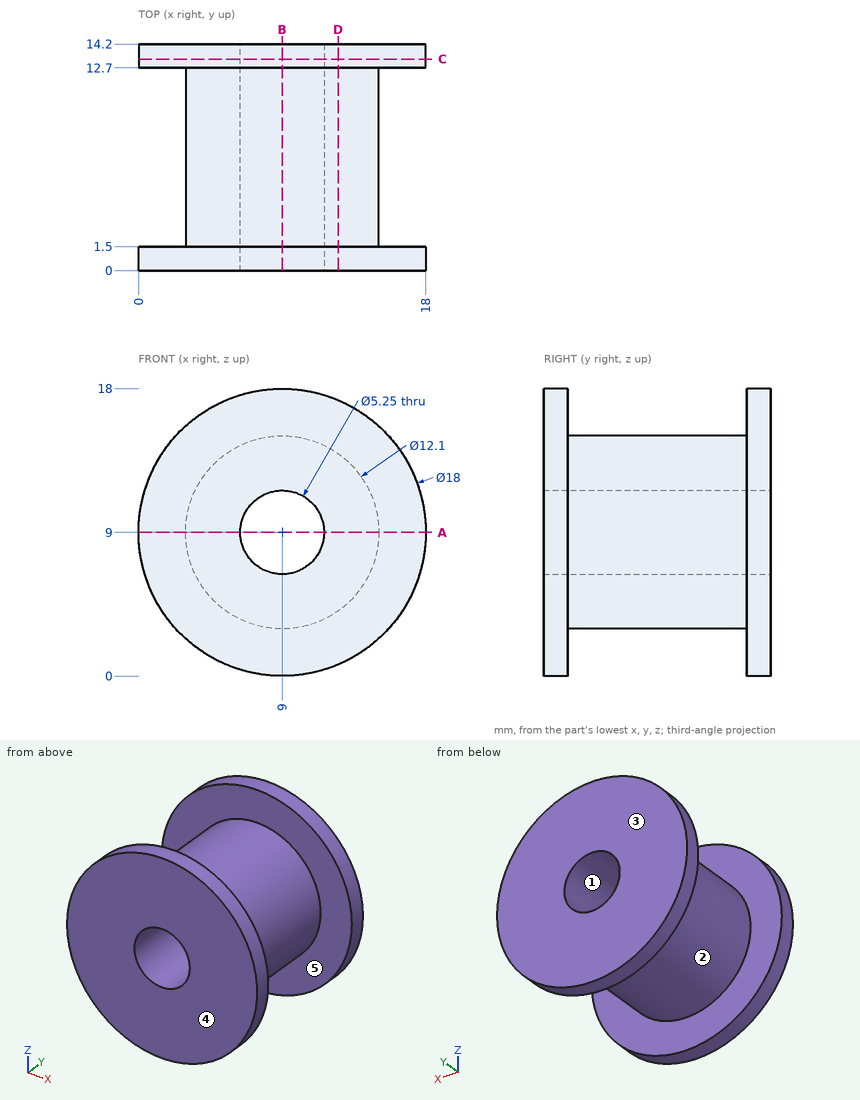
Verification items for this drawing (mm, ordinates from the low corner). A direction names the side the tool comes from. Give positions to 0.01 mm unless a question says otherwise; leave off trailing zeros. Loops run counter-clockwise (first coordinate to the right, second up) from the corner with the lowest first, then second, coordinate; pieces in that order, holes last. Notation, with made-up numbers: M -12.75,-24 L 3.25,-24 A26 cw 3.25,7 Z; hole C 54,43 d11. An arc over 180 degrees is marked long. Answer as a JSON object with one key per item and string values. Group by question number.
Q1. Access from +Z, -Z, +X, -X, +Y, -Y to the whole of each face (thin tool, end or side, straight path). Record for the marked faces 4 and 5.
Q2. Cross-section at B-B on x = 9. Record the cut outline in (y, z) (3 decimals), then the cut area to 3 significant figures.
Q3. Cross-section at D-D on x = 12.5. Record the cut outline in (y, z).
Q4. Cross-section at A-A on z = 9. Record the cut outline in (x, y) (3 decimals), then the cut area to 3 significant figures.
Q5. Go/stop test with flat-tipped pins: P1, Ø5.5, axis at x = 13, z = 6.5, coming from the -Y side; P2, Ø1, axis at x = 4, y = 12, coming from the -Z side; P3, Ø2, axis at y = 5, z = 4, coming from the -X side; P4, Ø4, axis at x = 5.5, y = 8.5, coming from the -Z side. Record where each tip stops, or that it passes through.
Q6. Cross-section at C-C on y = 13.25. Record the cut outline in (x, z) (3 decimals).
Q7. Material ranges on line 1 along X through (y, z) = (9.75, 9) (3 decimals); line 2 along Y through (x, z) = (1.5, 4.5), recorded low to high. Write a range as [from, to].
Q8. Release check for a two-part mould opening along Z. For the marked faces 1, 2 and 3 record: released by +Z, released by -Z, zero draft, split by the parting line, or undercut.
Evaluation:
{
 "1": {"face 4": "+Z, -Z, +X, -X, -Y", "face 5": "none"},
 "2": {"outline": "M 0,0 L 1.5,0 L 1.5,2.95 L 12.7,2.95 L 12.7,0 L 14.2,0 L 14.2,6.375 L 0,6.375 Z; M 0,11.625 L 14.2,11.625 L 14.2,18 L 12.7,18 L 12.7,15.05 L 1.5,15.05 L 1.5,18 L 0,18 Z", "area": "115 mm2"},
 "3": {"outline": "M 0,0.71 L 1.5,0.71 L 1.5,4.07 L 12.7,4.07 L 12.7,0.71 L 14.2,0.71 L 14.2,17.29 L 12.7,17.29 L 12.7,13.93 L 1.5,13.93 L 1.5,17.29 L 0,17.29 Z"},
 "4": {"outline": "M 0,0 L 6.375,0 L 6.375,14.2 L 0,14.2 L 0,12.7 L 2.95,12.7 L 2.95,1.5 L 0,1.5 Z; M 11.625,0 L 18,0 L 18,1.5 L 15.05,1.5 L 15.05,12.7 L 18,12.7 L 18,14.2 L 11.625,14.2 Z", "area": "115 mm2"},
 "5": {"P1": "stops at y = 0", "P2": "stops at z = 4.96", "P3": "stops at x = 4.46", "P4": "stops at z = 3.14"},
 "6": {"outline": "C 9,9 d18; hole C 9,9 d5.25"},
 "7": {"line 1": "x = [2.95, 6.375], [11.625, 15.05]", "line 2": "y = [0, 1.5], [12.7, 14.2]"},
 "8": {"face 1": "undercut", "face 2": "split by the parting line", "face 3": "zero draft"}
}
